The model under review builds one solid part; all positions refer to its coordinate system, in mm. Face numbers are marked on the shaded views. A direction names the side the tool comes from. Coordinates: 2 decimals unless noted, no trailing zeros. Loops run counter-clockwise (first coordinate to the right, second up) from the corner with the lowest first, then second, coordinate; pieces in that order, holes last. Notation, with made-up numbers: (-39, 4.25) - (-22, 4.25) arc R21 cw to (-22, 37.25) - close; hole circle Ø6 at (19, 63.5). An arc over 180 degrees is marked (long way). Use a Markdown table: item, result. Add a question column.
1) To check wall thickness, follow L1, parallel to X at y = 5.75, z = 2.7; L2, parallel to Y at x = -11.2, z = 0.45; L3, parallel to X at y = -4.25, z = 2.65. State the ranges of each line that lie inside material, in increasing order. Write a range as [from, to].
2) Add section A-A, the plane z = 2.15. Give the boundary of the cut face in (x, y).
3) The part is to be moulded in two halves that separate along Y. For the marked faces 1, 2 and 3, say which applies: pulls with the +Y half, pulls with the -Y half, needs draft (parallel to the pull), parting line crosses it, or undercut.
4) For the marked faces 4, 5 and 6, list the 3-axis set-ups (+Z, -Z, +X, -X, +Y, -Y) from which the entire face can be reached by the end or side of a thin tool; tool diameter is ignored.
5) Clearance check with a flat-ended pin moving along its axis: pin 1 (2.5 mm diameter, centred on x = -11.2, y = 0, fed in from +Z). State where the tip first meets the part, or that it passes through.
6) Add section C-C, the plane y = 0. Give the boundary of the cut face in (x, z), and give its area (3 significant figures).
7) Add section B-B, the plane x = -11.2. Give the boundary of the cut face in (y, z), and give its area (3 significant figures).
8) Add section D-D, the plane x = -7. Give the boundary of the cut face in (y, z), and give its area (3 significant figures).
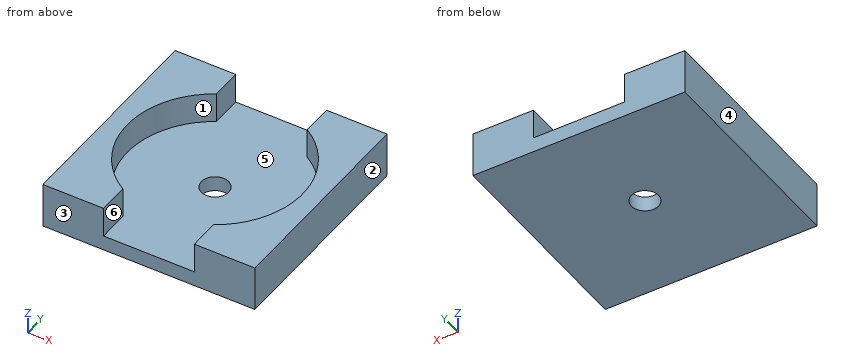
```python
from build123d import *

# Parameters (mm, degrees)
SKETCH006_W     = 14
SKETCH006_H     = 14
PAD002_DEPTH    = 3
POCKET004_DEPTH = 2
SKETCH008_R     = 0.9
POCKET005_DEPTH = 1.001


with BuildPart() as part:
    # Sketch006 → Pad002 (new body)
    with BuildSketch(Plane.XY):
        Rectangle(SKETCH006_W, SKETCH006_H)
    extrude(amount=PAD002_DEPTH)

    # Sketch007 (on Face6 of Pad002) → Pocket004 (cut)
    with BuildSketch(Plane.XY.offset(3)):
        with BuildLine():
            Line((-3, 7), (-3, 4.963869))
            ThreePointArc((-3, 4.963869), (-5.8, 0), (-3, -4.963869))
            Line((-3, -7), (-3, -4.963869))
            Line((3, -7), (-3, -7))
            Line((3, -4.963869), (3, -7))
            ThreePointArc((3, -4.963869), (5.8, 0), (3, 4.963869))
            Line((3, 7), (3, 4.963869))
            Line((-3, 7), (3, 7))
        make_face()
    extrude(amount=-POCKET004_DEPTH, mode=Mode.SUBTRACT)

    # Sketch008 (on Face6 of Pocket004) → Pocket005 (cut, through all)
    with BuildSketch(Plane.XY.offset(1)):
        Circle(SKETCH008_R)
    extrude(amount=-POCKET005_DEPTH, mode=Mode.SUBTRACT)


with BuildPart() as part_1:
    # Clone placement: moved
    add(part.part.moved(Location((-11.2, 0, 0))))


solid = part_1.part
```
From the geometry:
| question | item | result |
|---|---|---|
| 1 | L1 | x = [-18.2, -14.2], [-8.2, -4.2] |
| 1 | L2 | y = [-7, -0.9], [0.9, 7] |
| 1 | L3 | x = [-18.2, -15.15], [-7.25, -4.2] |
| 2 | outline | (-18.2, -7) - (-14.2, -7) - (-14.2, -4.96) arc R5.8 cw to (-14.2, 4.96) - (-14.2, 7) - (-18.2, 7) - close; (-8.2, -7) - (-4.2, -7) - (-4.2, 7) - (-8.2, 7) - (-8.2, 4.96) arc R5.8 cw to (-8.2, -4.96) - close |
| 3 | face 1 | undercut |
| 3 | face 2 | needs draft |
| 3 | face 3 | pulls with the -Y half |
| 4 | face 4 | +Z, -Z, -X, +Y, -Y |
| 4 | face 5 | +Z |
| 4 | face 6 | +Z, +Y, -Y |
| 5 | pin 1 | stops at z = 1 |
| 6 | outline | (-18.2, 0) - (-12.1, 0) - (-12.1, 1) - (-17, 1) - (-17, 3) - (-18.2, 3) - close; (-10.3, 0) - (-4.2, 0) - (-4.2, 3) - (-5.4, 3) - (-5.4, 1) - (-10.3, 1) - close |
| 6 | area | 17.0 mm^2 |
| 7 | outline | (-7, 0) - (-0.9, 0) - (-0.9, 1) - (-7, 1) - close; (0.9, 0) - (7, 0) - (7, 1) - (0.9, 1) - close |
| 7 | area | 12.2 mm^2 |
| 8 | outline | (-7, 0) - (7, 0) - (7, 3) - (4, 3) - (4, 1) - (-4, 1) - (-4, 3) - (-7, 3) - close |
| 8 | area | 26.0 mm^2 |
